from build123d import *

# Parameters (mm, degrees)
F0_W     = 101.6
F0_H     = 152.4
F1_DEPTH = 76.2
F2_W     = 76.2
F2_H     = 25.4
F3_DEPTH = 50.8
F4_R     = 5.08


with BuildPart() as f1:
    # F0 (on Front) → F1 (new body)
    with BuildSketch(Plane.XZ):
        with Locations((34.750886, -17.486643)):
            Rectangle(F0_W, F0_H)
    extrude(amount=F1_DEPTH)

    # F2 (on face) → F3 (cut)
    with BuildSketch(Plane.XZ.offset(76.2)):
        with Locations((34.750886, 35.853357)):
            Rectangle(F2_W, F2_H)
        with Locations((34.750886, 0.293357)):
            Rectangle(F2_W, F2_H)
        with Locations((34.750886, -35.266643)):
            Rectangle(F2_W, F2_H)
        with Locations((34.750886, -70.826643)):
            Rectangle(F2_W, F2_H)
    extrude(amount=-F3_DEPTH, mode=Mode.SUBTRACT)

    # F4
    f4_edges = [f1.edges().sort_by_distance(p)[0] for p in [
        (34.750886, -76.2, 58.713357),
        (85.550886, -38.1, 58.713357),
        (85.550886, -38.1, -93.686643),
        (-16.049114, -38.1, -93.686643),
        (-16.049114, -38.1, 58.713357),
        (85.550886, -76.2, -17.486643),
    ]]
    fillet(f4_edges, radius=F4_R)


solid = f1.part
Build history of the part. All positions in model axes, mm. A direction names the side the tool comes from. Give positions to 0.01 mm unless a question says otherwise; leave off trailing zeros. Order: outer loops, then holes, each group sorted by start corner. A loop starts at its lowest first (then second) coordinate and runs counter-clockwise, first axis right, second up. Notation, with made-up numbers: M 84,-38 L 118,-38 A16 ccw 118,-18 Z; hole C 4.5,24.5 d6. An arc over 180 degrees is marked long. Put each result on its own line as item: value.
Item 1: Drop a flat-ended pin along its axis: pin 1 Ø8 at (x, z) = (28.5, -67) entering from -Y. Give the stop position or say it passes through.
Results are:
pin 1: y = -25.4
Item 2: Cut at B-B on z = 27. Write the cut outline in (x, y).
Results are:
outline: M -16.05,-76.2 L -3.35,-76.2 L -3.35,-25.4 L 72.85,-25.4 L 72.85,-76.2 L 80.47,-76.2 A5.08 ccw 85.55,-71.12 L 85.55,0 L -16.05,0 Z
Item 3: Pull direction X, two halves, no side cores. Call faces 3 (the face through (32, -76.2, -19)), 4 (the face through (-14.6, -38.633, 57.186)), 5 (the face through (72.851, -51, 36)): +X half, -X half, draft (parallel to the pull), parting line (faces both ways), or undercut.
Results are:
face 3: draft
face 4: -X half
face 5: undercut
Item 4: Which spindle directions (+Z, -Z, +X, -X, +Y, -Y) get a long thin tool onto all of the face, cutting with end or side? Do faces 1 (the face through (34, -51, -58.127)), 2 (the face through (-14.6, -38.63, -92.16)). Say none if no direction does.
Results are:
face 1: -Y
face 2: -Z, -X, +Y, -Y
Item 5: Cut at C-C on x = 67. Write the cut outline in (y, z), then the cut area to 3 significant figures.
Results are:
outline: M -76.2,-93.69 L 0,-93.69 L 0,58.71 L -71.12,58.71 A5.08 ccw -76.2,53.63 L -76.2,48.55 L -25.4,48.55 L -25.4,23.15 L -76.2,23.15 L -76.2,12.99 L -25.4,12.99 L -25.4,-12.41 L -76.2,-12.41 L -76.2,-22.57 L -25.4,-22.57 L -25.4,-47.97 L -76.2,-47.97 L -76.2,-58.13 L -25.4,-58.13 L -25.4,-83.53 L -76.2,-83.53 Z
area: 6,450 mm2
Item 6: Wall check: probe 1 along Z at (x, y) = (12.5, -27.5); probe 2 along X at (y, z) = (-44, 45); probe 3 along Y at (x, z) = (52, 30). Give the ranges that are in metal, low to high.
Results are:
probe 1: -93.69 to -83.53, -58.13 to -47.97, -22.57 to -12.41, 12.99 to 23.15, 48.55 to 58.71
probe 2: -16.05 to -3.35, 72.85 to 85.55
probe 3: -25.4 to 0
Item 7: Cut at A-A on y = -48.5. Write the cut outline in (x, z), then the cut area to 3 significant figures.
Results are:
outline: M -16.05,-88.61 A5.08 ccw -10.97,-93.69 L 80.47,-93.69 A5.08 ccw 85.55,-88.61 L 85.55,53.63 A5.08 ccw 80.47,58.71 L -10.97,58.71 A5.08 ccw -16.05,53.63 Z; hole M -3.35,-83.53 L 72.85,-83.53 L 72.85,-58.13 L -3.35,-58.13 Z; hole M -3.35,-47.97 L 72.85,-47.97 L 72.85,-22.57 L -3.35,-22.57 Z; hole M -3.35,-12.41 L 72.85,-12.41 L 72.85,12.99 L -3.35,12.99 Z; hole M -3.35,23.15 L 72.85,23.15 L 72.85,48.55 L -3.35,48.55 Z
area: 7,720 mm2
